```python
from build123d import *

# Parameters (mm, degrees)
F1_DEPTH  = 38
F2_R      = 20.15
F3_DEPTH  = 26
F5_DEPTH  = 93
F7_DEPTH  = 12.5
F8_R      = 15
F9_DEPTH  = 3.2
F10_R     = 15.7
F11_DEPTH = 1.3
F12_R     = 15
F13_DEPTH = 14
F14_R     = 12.8
F15_DEPTH = 16.001
F17_DEPTH = 4
F19_D     = 5.5
F19_DEPTH = 8.2
F19_TIP   = 1.6523667023
F21_DEPTH = 4
F23_D     = 5.5
F23_DEPTH = 8.2
F23_TIP   = 1.6523667023


with BuildPart() as f1:
    # F0 (on Top) → F1 (new body)
    with BuildSketch(Plane.XY):
        with BuildLine():
            ThreePointArc((8.1700673192, 21.5), (0, 23), (-8.1700673192, 21.5))
            ThreePointArc((-8.1700673192, 21.5), (-16.2634559673, 16.2634559673), (-21.5, 8.1700673192))
            Line((-21.5, 8.1700673192), (-21.5, -8.1700673192))
            ThreePointArc((-21.5, -8.1700673192), (-16.2634559673, -16.2634559673), (-8.1700673192, -21.5))
            ThreePointArc((-8.1700673192, -21.5), (0, -23), (8.1700673192, -21.5))
            ThreePointArc((8.1700673192, -21.5), (16.2634559673, -16.2634559673), (21.5, -8.1700673192))
            Line((21.5, -8.1700673192), (21.5, 8.1700673192))
            ThreePointArc((21.5, 8.1700673192), (16.2634559673, 16.2634559673), (8.1700673192, 21.5))
        make_face()
    extrude(amount=F1_DEPTH)

    # F2 (on Top) → F3 (cut)
    with BuildSketch(Plane.XY):
        Circle(F2_R)
    extrude(amount=F3_DEPTH, mode=Mode.SUBTRACT)

    # F4 (on face) → F5 (join)
    with BuildSketch(Plane.XY.offset(38)):
        with BuildLine():
            Line((15.748015748, 11.5), (-15.748015748, 11.5))
            ThreePointArc((-15.748015748, 11.5), (-19.5, 0), (-15.748015748, -11.5))
            Line((-15.748015748, -11.5), (15.748015748, -11.5))
            ThreePointArc((15.748015748, -11.5), (19.5, 0), (15.748015748, 11.5))
        make_face()
    extrude(amount=F5_DEPTH)

    # F6 (on Front) → F7 (cut, symmetric)
    with BuildSketch(Plane.XZ):
        with BuildLine():
            ThreePointArc((-22.9993669171, 108.1706499767), (-1.4508057769, 130.9541970584), (22.7948567954, 111.0650454609))
            Line((22.7948567954, 111.0650454609), (28.0992928892, 135.5375498533))
            Line((28.0992928892, 135.5375498533), (-36.6138778627, 135.5375498533))
            Line((-36.6138778627, 135.5375498533), (-22.9993669171, 108.1706499767))
        make_face()
    extrude(amount=F7_DEPTH, both=True, mode=Mode.SUBTRACT)

    # F8 (on face) → F9 (cut)
    with BuildSketch(Plane(origin=(0, 11.5, 0), x_dir=(-1, 0, 0), z_dir=(0, 1, 0))):
        with Locations((0, 108)):
            Circle(F8_R)
    extrude(amount=-F9_DEPTH, mode=Mode.SUBTRACT)

    # F10 (on face) → F11 (cut)
    with BuildSketch(Plane(origin=(0, 8.3, 0), x_dir=(-1, 0, 0), z_dir=(0, 1, 0))):
        with Locations((0, 108)):
            Circle(F10_R)
    extrude(amount=-F11_DEPTH, mode=Mode.SUBTRACT)

    # F12 (on face) → F13 (cut)
    with BuildSketch(Plane(origin=(0, 7, 0), x_dir=(-1, 0, 0), z_dir=(0, 1, 0))):
        with Locations((0, 108)):
            Circle(F12_R)
    extrude(amount=-F13_DEPTH, mode=Mode.SUBTRACT)

    # F14 (on face) → F15 (cut, through all)
    with BuildSketch(Plane(origin=(0, -7, 0), x_dir=(-1, 0, 0), z_dir=(0, 1, 0))):
        with Locations((0, 108)):
            Circle(F14_R)
    extrude(amount=-F15_DEPTH, mode=Mode.SUBTRACT)

    # F16 (on face) → F17 (cut)
    with BuildSketch(Plane.YZ.offset(21.5)):
        with BuildLine():
            Line((5.5, 36), (-5.5, 36))
            ThreePointArc((-5.5, 36), (-6.9142135624, 35.4142135624), (-7.5, 34))
            Line((-7.5, 34), (-7.5, 30))
            ThreePointArc((-7.5, 30), (-6.9142135624, 28.5857864376), (-5.5, 28))
            Line((-5.5, 28), (5.5, 28))
            ThreePointArc((5.5, 28), (6.9142135624, 28.5857864376), (7.5, 30))
            Line((7.5, 30), (7.5, 34))
            ThreePointArc((7.5, 34), (6.9142135624, 35.4142135624), (5.5, 36))
        make_face()
    extrude(amount=-F17_DEPTH, mode=Mode.SUBTRACT)

    # F19
    with Locations(Plane.YZ.offset(17.5)):
        with Locations((0, 32)):
            Hole(F19_D / 2, depth=F19_DEPTH)
            with Locations((0, 0, -(F19_DEPTH + F19_TIP / 2))):  # 118° drill point
                Cone(0, F19_D / 2, F19_TIP, mode=Mode.SUBTRACT)

    # F20 (on face) → F21 (cut)
    with BuildSketch(Plane(origin=(-21.5, 0, 0), x_dir=(0, -1, 0), z_dir=(-1, 0, 0))):
        with BuildLine():
            Line((5.5, 36), (-5.5, 36))
            ThreePointArc((-5.5, 36), (-6.9142135624, 35.4142135624), (-7.5, 34))
            Line((-7.5, 34), (-7.5, 30))
            ThreePointArc((-7.5, 30), (-6.9142135624, 28.5857864376), (-5.5, 28))
            Line((-5.5, 28), (5.5, 28))
            ThreePointArc((5.5, 28), (6.9142135624, 28.5857864376), (7.5, 30))
            Line((7.5, 30), (7.5, 34))
            ThreePointArc((7.5, 34), (6.9142135624, 35.4142135624), (5.5, 36))
        make_face()
    extrude(amount=-F21_DEPTH, mode=Mode.SUBTRACT)

    # F23
    with Locations(Plane(origin=(-17.5, 0, 0), x_dir=(0, -1, 0), z_dir=(-1, 0, 0))):
        with Locations((0, 32)):
            Hole(F23_D / 2, depth=F23_DEPTH)
            with Locations((0, 0, -(F23_DEPTH + F23_TIP / 2))):  # 118° drill point
                Cone(0, F23_D / 2, F23_TIP, mode=Mode.SUBTRACT)


solid = f1.part
```
Here's how the part is built. I have some questions about the finished solid (model axes, mm). A direction names the side the tool comes from. Give positions to 0.01 mm unless a question says otherwise; leave off trailing zeros. Write each loop counter-clockwise with the first axis right and the second up, starting at its lowest first coordinate (ties: lowest second). Pieces come first, ordered by that corner, then holes.
(1) Imagine slicing it at B-B, the plane z = 96.5. Write out the boundary of the cut face in (x, y).
Output values:
outline: (-15.75, -11.5) - (-5.62, -11.5) - (-5.62, -7) - (-9.63, -7) - (-9.63, 7) - (-10.69, 7) - (-10.69, 8.3) - (-9.63, 8.3) - (-9.63, 11.5) - (-15.75, 11.5) arc R19.5 ccw to start; (5.62, -11.5) - (15.75, -11.5) arc R19.5 ccw to (15.75, 11.5) - (9.63, 11.5) - (9.63, 8.3) - (10.69, 8.3) - (10.69, 7) - (9.63, 7) - (9.63, -7) - (5.62, -7) - close
(2) Imagine slicing it at C-C, the plane y = -15. Write out the boundary of the cut face in (x, z).
Output values:
outline: (-17.44, 0) - (-13.45, 0) - (-13.45, 26) - (13.45, 26) - (13.45, 0) - (17.44, 0) - (17.44, 38) - (-17.44, 38) - close
(3) Thinking about a two-plate mould opening in X: for faces 1 (the face through (20, 7.5, 32)), 2 (the face through (2.044, 7.659, 123.566)), 3 (the face through (7.935, -0.104, 31.534)), 4 (the face through (-17.5, -2, 29)), which applies, pulls with the +X half, pulls with the -X half, needs draft (parallel to the pull), parting line crosses it, or undercut?
Output values:
face 1: needs draft
face 2: undercut
face 3: pulls with the +X half
face 4: pulls with the -X half
(4) On a 3-axis mill with a long thin cutter (end or side, diameter ignored), from which of +Z, -Z, +X, -X, +Y, -Y can I reach the whole of each face in a straight line? I mean faces 5 (the face through (-11, -7, 115)), 6 (the face through (0, -11.5, 74)), 7 (the face through (-20, 7.5, 32)), 8 (the face through (0, 11.5, 74)). Say none if no direction works.
Output values:
face 5: +Y
face 6: +Z, +X, -X, -Y
face 7: -X
face 8: +Z, +X, -X, +Y
(5) Will these pins go through, and if not, where does the flat tip stop? pin 1 (1.2 mm diameter, centred on x = -19, z = 32.5, fed in from -Y); pin 2 (12 mm diameter, centred on x = -8, y = 11, fed in from +Z); pin 3 (15.5 mm diameter, centred on x = 8, z = 72.5, fed in from +Y); pin 4 (24 mm diameter, centred on x = 0, z = 108, fed in from +Y).
Output values:
pin 1: stops at y = -13.8
pin 2: stops at z = 130.91
pin 3: stops at y = 11.5
pin 4: passes through
(6) Imagine slicing it at A-A, the plane x = 0. Write out the boundary of the cut face in (y, z).
Output values:
outline: (-23, 0) - (-20.15, 0) - (-20.15, 26) - (20.15, 26) - (20.15, 0) - (23, 0) - (23, 38) - (11.5, 38) - (11.5, 93) - (8.3, 93) - (8.3, 92.3) - (7, 92.3) - (7, 93) - (-7, 93) - (-7, 95.2) - (-11.5, 95.2) - (-11.5, 38) - (-23, 38) - close; (-11.5, 120.8) - (-7, 120.8) - (-7, 123) - (7, 123) - (7, 123.7) - (8.3, 123.7) - (8.3, 123) - (11.5, 123) - (11.5, 131) - (-11.5, 131) - close
(7) If I drill on L1, parallel to Z at x = 0, y = 8; L2, parallel to Z at x = 0, y = 9; L3, parallel to Z at x = 11, y = 13, over which ranges is the centre line in solid material (lowest first)?
Output values:
L1: z = 26 to 92.3, 123.7 to 131
L2: z = 26 to 93, 123 to 131
L3: z = 26 to 38
